Read the model definition and answer for the solid it produces. Units are mm, in the model's axes. Face numbers are marked on the shaded views. A direction names the side the tool comes from. Round coordinates to 2 decimals unless told otherwise and drop trailing zeros. Write each loop counter-clockwise with the first axis right and the second up, starting at its lowest first coordinate (ties: lowest second). Pieces come first, ordered by that corner, then holes. Notation, with made-up numbers: (-14.75, -32) - (29.25, -32) arc R22 cw to (29.25, -22) - close; hole circle Ø6 at (-33, 4.25). An arc over 180 degrees is marked (long way). Use one line per item in the form item = value. Start each with the question number.
1) The part is cut by section D-D, the plane y = -1.5. Give the vertices of the cut face in (x, z), plus the area to 3 significant figures.
2) For a pull along X with two mould halves and no side action, classify the marked faces 3, 4 and 5 as released by +X, released by -X, zero draft, split by the parting line, or undercut.
3) Consider line 1 along Z through (x, y) = (0, -6); line 2 along X through (y, z) = (-5.75, -2.5); line 3 along Y through (x, z) = (-4.25, -1.75). Determine where each line is inside the solid, lowest interval first. Write a range as from..to.
4) The part is cut by section C-C, the plane y = -7.5. Give the vertices of the cut face in (x, z).
5) For the marked faces 1 and 2, determine the directions among +Z, -Z, +X, -X, +Y, -Y from which every point of the face is accessible in a straight line to the end or side of a thin tool.
6) Each of these flat-tipped pins is pushed along its axis until it touches: pin 1 (1.5 mm diameter, centred on y = -10, z = -6.5, fed in from +X); pin 2 (5.5 mm diameter, centred on x = 2, z = -0.5, fed in from -Y); pin 3 (2 mm diameter, centred on y = -8, z = 7, fed in from -X). Where does it stop, or does it pass through?
from build123d import *

# Parameters (mm, degrees)
F0_R     = 9
F1_DEPTH = 12
F2_R     = 9
F2_R_2   = 7
F3_DEPTH = 10
F4_R     = 5.5
F5_DEPTH = 10
F6_R     = 1.99999


# Not quite as in the source:
# - a fillet or chamfer is up to 0.001 mm smaller than in the source, because OpenCascade refuses the exact size


with BuildPart() as f1:
    # F0 (on Front) → F1 (new body)
    with BuildSketch(Plane.XZ):
        Circle(F0_R)
    extrude(amount=F1_DEPTH)

    # F2 (on face) → F3 (cut)
    with BuildSketch(Plane.XZ.offset(12)):
        Circle(F2_R)
        Circle(F2_R_2, mode=Mode.SUBTRACT)
    extrude(amount=-F3_DEPTH, mode=Mode.SUBTRACT)

    # F4 (on face) → F5 (cut)
    with BuildSketch(Plane.XZ.offset(12)):
        Circle(F4_R)
    extrude(amount=-F5_DEPTH, mode=Mode.SUBTRACT)

    # F6 (radius 2 in the source; OpenCascade refuses exactly that, so slightly less here)
    f6_edges = [f1.edges().sort_by_distance(p)[0] for p in [
        (-9, 0, 0),
    ]]
    fillet(f6_edges, radius=F6_R)


solid = f1.part
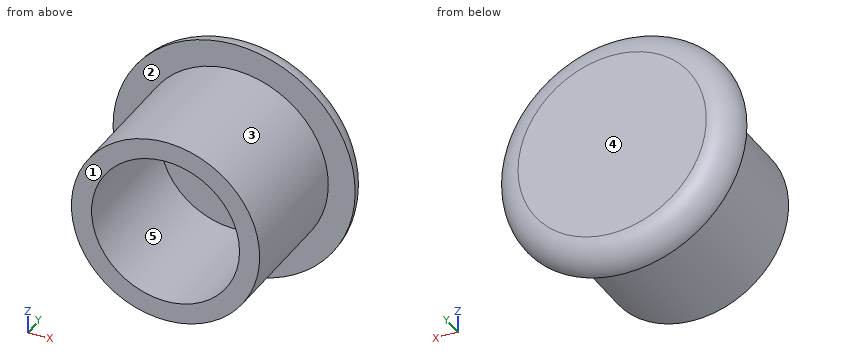
Geometry results:
q1.outline = circle Ø17.87 at (0, 0)
q1.area = 251 mm2
q2.face_3 = split by the parting line
q2.face_4 = zero draft
q2.face_5 = undercut
q3.line_1 = -7..-5.5, 5.5..7
q3.line_2 = -6.54..-4.9, 4.9..6.54
q3.line_3 = -2..0
q4.outline = circle Ø14 at (0, 0); hole circle Ø11 at (0, 0)
q5.face_1 = +Z, -Z, +X, -X, -Y
q5.face_2 = -Y
q6.pin_1 = 3.99
q6.pin_2 = -2
q6.pin_3 = -3.61
